```python
from build123d import *

# Parameters (mm, degrees)
PROFILE_EXTRUDE_DEPTH                           = 31.75
INTERIOR_START                                  = -3
INTERIOR_SKETCH_W                               = 57.5
INTERIOR_SKETCH_H                               = 37.4
INTERIOR_CUT_DEPTH                              = 50
OPENING_CUT_REACH                               = 77.925
OPENING_SKETCH_W                                = 47.5
OPENING_SKETCH_H                                = 27.4
CHAMFER1_SIZE                                   = 5
FILLET1_R                                       = 1
CUT_EXTRUDE3_REACH                              = 77.925
SKETCH5_R                                       = 9.5
FILLET2_R                                       = 1.5
FILLET3_R                                       = 4
CSK_FOR_M3_FLAT_HEAD_MACHINE_SCREW1_D           = 3.6
CSK_FOR_M3_FLAT_HEAD_MACHINE_SCREW1_CSINK_D     = 9.8
CSK_FOR_M3_FLAT_HEAD_MACHINE_SCREW1_CSINK_ANGLE = 90


with BuildPart() as part:
    # Profile Sketch → Profile Extrude (new, symmetric)
    with BuildSketch(Plane(origin=(0, 0, 0), x_dir=(0, 0, -1), z_dir=(1, 0, 0))):
        Polygon((0, 0), (0, 43.6), (-20, 43.6), (-20, 53.6), (43.4, 53.6), (43.4, 0), align=None)
    extrude(amount=PROFILE_EXTRUDE_DEPTH, both=True)

    # Interior Sketch → Interior Cut (cut)
    with BuildSketch(Plane.XZ.offset(INTERIOR_START)):
        with Locations((0, -21.7)):
            Rectangle(INTERIOR_SKETCH_W, INTERIOR_SKETCH_H)
    extrude(amount=-INTERIOR_CUT_DEPTH, mode=Mode.SUBTRACT)

    # Opening Sketch → Opening Cut (cut, up to next)
    with BuildSketch(Plane(origin=(0, 53.6, 0), x_dir=(1, 0, 0), z_dir=(0, 1, 0)), mode=Mode.PRIVATE) as opening_cut_sk1:
        with Locations((0, 21.7)):
            Rectangle(OPENING_SKETCH_W, OPENING_SKETCH_H)
    opening_cut_tool1 = extrude(opening_cut_sk1.sketch, amount=-OPENING_CUT_REACH, mode=Mode.PRIVATE) & part.part
    add(opening_cut_tool1.solids().sort_by_distance((0, 53.6, -21.7))[0], mode=Mode.SUBTRACT)

    # Chamfer1
    chamfer1_edges = [part.edges().sort_by_distance(p)[0] for p in [
        (0, 53, -3),
        (28.75, 53, -21.7),
        (0, 53, -40.4),
        (-28.75, 53, -21.7),
    ]]
    chamfer(chamfer1_edges, length=CHAMFER1_SIZE - 0.0001)  # a hair under: the kernel refuses the full size

    # Fillet1
    fillet1_edges = [part.edges().sort_by_distance(p)[0] for p in [
        (28.75, 25.50005, -40.4),
        (28.75, 25.50005, -3),
        (-28.75, 25.50005, -40.4),
        (-28.75, 25.50005, -3),
    ]]
    fillet(fillet1_edges, radius=FILLET1_R)

    # Sketch5 → Cut-Extrude3 (cut, up to next)
    with BuildSketch(Plane.XZ, mode=Mode.PRIVATE) as cut_extrude3_sk1:
        with Locations(Location((0, -21.7, 0), (0, 0, 270))):
            Circle(SKETCH5_R)
    cut_extrude3_tool1 = extrude(cut_extrude3_sk1.sketch, amount=-CUT_EXTRUDE3_REACH, mode=Mode.PRIVATE) & part.part
    add(cut_extrude3_tool1.solids().sort_by_distance((0, 0, -21.7))[0], mode=Mode.SUBTRACT)

    # Fillet2
    fillet2_edges = [part.edges().sort_by_distance(p)[0] for p in [
        (0, 0, -12.2),
        (0, 3, -12.2),
    ]]
    fillet(fillet2_edges, radius=FILLET2_R - 0.0001)  # a hair under: the kernel refuses the full size

    # Fillet3
    fillet3_edges = [part.edges().sort_by_distance(p)[0] for p in [
        (0, 0, 0),
        (0, 53.6, 20),
        (0, 53.6, -43.4),
        (0, 0, -43.4),
        (31.75, 53.6, -11.7),
        (31.75, 48.6, 20),
        (31.75, 21.8, 0),
        (31.75, 0, -21.7),
        (-31.75, 21.8, 0),
        (-31.75, 48.6, 20),
        (-31.75, 53.6, -11.7),
        (-31.75, 26.8, -43.4),
        (-31.75, 0, -21.7),
        (31.75, 26.8, -43.4),
    ]]
    fillet(fillet3_edges, radius=FILLET3_R)

    # CSK for M3 Flat Head Machine Screw1 (through all)
    with Locations(Plane(origin=(-17.75, 53.6, 10), x_dir=(0, 0, 1), z_dir=(0, 1, 0))):
        with Locations((0, 0), (0, 35.5)):
            CounterSinkHole(CSK_FOR_M3_FLAT_HEAD_MACHINE_SCREW1_D / 2, CSK_FOR_M3_FLAT_HEAD_MACHINE_SCREW1_CSINK_D / 2, counter_sink_angle=CSK_FOR_M3_FLAT_HEAD_MACHINE_SCREW1_CSINK_ANGLE)


solid = part.part
```
Model file for the job. Use its own axes, mm. A direction names the side the tool comes from. Round coordinates to 2 decimals unless told otherwise and drop trailing zeros. Loops run counter-clockwise (first coordinate to the right, second up) from the corner with the lowest first, then second, coordinate; pieces in that order, holes last. Notation, with made-up numbers: M 65,16.25 L 78,16.25 A25 cw 78,37.25 Z; hole C 50.25,-3.75 d8. An arc over 180 degrees is marked long. Put each result on its own line as item: value. Start each with the question number.
Item 1: Drop flat-ended pins along their axis: P1, Ø10, axis at y = 25, z = 3, coming from the +X side; P2, Ø0.5, axis at x = -9, y = 53.5, coming from the +Z side; P3, Ø4.5, axis at x = 17.75, z = 10, coming from the -Y side; P4, Ø15, axis at x = 0, z = -21.7, coming from the -Y side. Give the stop position or say it passes through.
Item 2: Mould opens along X. For faces 1 (the face through (0, 25, -3)), 2 (the face through (31.75, 27, -18)), 3 (the face through (0, 24, 0)) say: released by +X, released by -X, zero draft, split by the parting line, or undercut.
Item 3: Drill centre lines: line 1 along X through (y, z) = (47.5, 10); line 2 along Z through (x, y) = (-17.75, 46.25); line 3 along Z through (x, y) = (7, 37.5). Where is each one in solid material? Low to high.
Item 4: 3-axis set-ups, long thin cutter, end or side, ignore diameter. For faces 4 (the face through (-30.609, 24.077, -1.203)), 5 (the face through (0, 50, -5)), 6 (the face through (0, 47, 20)): which of +Z, -Z, +X, -X, +Y, -Y reach the whole face in a straight line?
Item 5: Cut at A-A (z = 10). List the corners of the cut face in (x, y).
Item 6: Cut at C-C (y = 9). List the corners of the cut face in (x, z), then the cut area to 3 significant figures.
Answer block:
1. P1: x = 31.21
1. P2: z = 17.64
1. P3: y = 43.6
1. P4: through
2. face 1: undercut
2. face 2: released by +X
2. face 3: zero draft
3. line 1: -31.75 to -19.55, -15.95 to 15.95, 19.55 to 31.75
3. line 2: -43.4 to -40.4, -3 to 8.2, 11.8 to 20
3. line 3: -43.4 to -40.4, -3 to 0
4. face 4: +Z, -X, -Y
4. face 5: none
4. face 6: +Z, +X, -X, +Y, -Y
5. outline: M -31.75,43.6 L -19.55,43.6 L -19.55,50.5 L -22.65,53.6 L -27.75,53.6 A4 ccw -31.75,49.6 Z; M -15.95,43.6 L 15.95,43.6 L 15.95,50.5 L 12.85,53.6 L -12.85,53.6 L -15.95,50.5 Z; M 19.55,43.6 L 31.75,43.6 L 31.75,49.6 A4 ccw 27.75,53.6 L 22.65,53.6 L 19.55,50.5 Z
6. outline: M -31.75,-39.4 A4 ccw -27.75,-43.4 L 27.75,-43.4 A4 ccw 31.75,-39.4 L 31.75,-4 A4 ccw 27.75,0 L -27.75,0 A4 ccw -31.75,-4 Z; hole M -28.75,-39.4 A1 ccw -27.75,-40.4 L 27.75,-40.4 A1 ccw 28.75,-39.4 L 28.75,-4 A1 ccw 27.75,-3 L -27.75,-3 A1 ccw -28.75,-4 Z
6. area: 593 mm2
